```python
from build123d import *

# Parameters (mm, degrees)
SKETCH1_W           = 77.47
SKETCH1_H           = 52.07
SKETCH1_R           = 1.5875
SKETCH1_H_2         = 52.34
BOSS_EXTRUDE3_DEPTH = 6.35
SKETCH2_W           = 19.05
SKETCH2_H           = 1
CUT_EXTRUDE1_DEPTH  = 193.995155978
SKETCH4_W           = 19.05
SKETCH4_H           = 1
CUT_EXTRUDE2_DEPTH  = 193.995155978
SKETCH5_W           = 257.81
SKETCH5_H           = 1
BOSS_EXTRUDE4_DEPTH = 215.9
SKETCH6_W           = 57.15
SKETCH6_H           = 31.75
CUT_EXTRUDE3_DEPTH  = 193.964841955
CUT_EXTRUDE5_DEPTH  = 193.995155978


with BuildPart() as part:
    # Sketch1 → Boss-Extrude3 (new body)
    with BuildSketch(Plane(origin=(0, 0, 0), x_dir=(1, 0, 0), z_dir=(0, 1, 0))):
        Polygon((148.59, 94.11025641), (129.54, 94.11025641), (129.54, 113.16025641), (-137.02974359, 113.16025641), (-137.02974359, 93.98), (-156.21, 93.98), (-156.21, -88.9), (-137.16, -88.9), (-137.16, -106.95), (-156.21, -106.95), (-156.21, -107.95), (148.59, -107.95), (148.59, -106.95), (129.54, -106.95), (129.54, -88.9), (148.59, -88.9), align=None)
        with Locations((-95.885, -80.915)):
            Rectangle(SKETCH1_W, SKETCH1_H, mode=Mode.SUBTRACT)
        with Locations((-5.715, -80.915)):
            Rectangle(SKETCH1_W, SKETCH1_H, mode=Mode.SUBTRACT)
        with Locations((84.455, -80.915)):
            Rectangle(SKETCH1_W, SKETCH1_H, mode=Mode.SUBTRACT)
        with Locations((84.455, 82.915)):
            Rectangle(SKETCH1_W, SKETCH1_H, mode=Mode.SUBTRACT)
        with Locations((84.455, 28.305)):
            Rectangle(SKETCH1_W, SKETCH1_H, mode=Mode.SUBTRACT)
        with Locations((84.455, -26.305)):
            Rectangle(SKETCH1_W, SKETCH1_H, mode=Mode.SUBTRACT)
        with Locations(Location((139.065, 75.334869264, 0), (0, 0, 270))):
            Circle(SKETCH1_R, mode=Mode.SUBTRACT)
        with Locations(Location((139.065, 80.910552749, 0), (0, 0, 270))):
            Circle(SKETCH1_R, mode=Mode.SUBTRACT)
        with Locations(Location((139.065, 86.618990604, 0), (0, 0, 270))):
            Circle(SKETCH1_R, mode=Mode.SUBTRACT)
        with Locations((-5.715, 82.915)):
            Rectangle(SKETCH1_W, SKETCH1_H, mode=Mode.SUBTRACT)
        with Locations((-95.885, -26.305)):
            Rectangle(SKETCH1_W, SKETCH1_H, mode=Mode.SUBTRACT)
        with Locations((-5.715, -26.17)):
            Rectangle(SKETCH1_W, SKETCH1_H_2, mode=Mode.SUBTRACT)
        with Locations((-95.885, 28.305)):
            Rectangle(SKETCH1_W, SKETCH1_H, mode=Mode.SUBTRACT)
        with Locations((-5.715, 28.305)):
            Rectangle(SKETCH1_W, SKETCH1_H, mode=Mode.SUBTRACT)
        with Locations((-95.885, 82.915)):
            Rectangle(SKETCH1_W, SKETCH1_H, mode=Mode.SUBTRACT)
    extrude(amount=BOSS_EXTRUDE3_DEPTH)

    # Sketch2 → Cut-Extrude1 (cut, through all)
    with BuildSketch(Plane(origin=(0, 6.35, 0), x_dir=(1, 0, 0), z_dir=(0, 1, 0))):
        with Locations((139.065, -107.45)):
            Rectangle(SKETCH2_W, SKETCH2_H)
    extrude(amount=-CUT_EXTRUDE1_DEPTH, mode=Mode.SUBTRACT)

    # Sketch4 → Cut-Extrude2 (cut, through all)
    with BuildSketch(Plane(origin=(0, 6.35, 0), x_dir=(1, 0, 0), z_dir=(0, 1, 0))):
        with Locations((-146.685, -107.45)):
            Rectangle(SKETCH4_W, SKETCH4_H)
    extrude(amount=-CUT_EXTRUDE2_DEPTH, mode=Mode.SUBTRACT)

    # Sketch5 → Boss-Extrude4 (add)
    with BuildSketch(Plane.XY.offset(-108.95)):
        with Locations((-5.715, 0.5)):
            Rectangle(SKETCH5_W, SKETCH5_H)
    extrude(amount=BOSS_EXTRUDE4_DEPTH)

    # Sketch6 → Cut-Extrude3 (cut, through all)
    with BuildSketch(Plane(origin=(0, 1, 0), x_dir=(1, 0, 0), z_dir=(0, 1, 0))):
        with Locations((-95.885, 82.915)):
            Rectangle(SKETCH6_W, SKETCH6_H)
        with Locations((-95.885, 28.305)):
            Rectangle(SKETCH6_W, SKETCH6_H)
        with Locations((-95.885, -26.305)):
            Rectangle(SKETCH6_W, SKETCH6_H)
        with Locations((-95.885, -80.915)):
            Rectangle(SKETCH6_W, SKETCH6_H)
        with Locations((-5.715, 82.915)):
            Rectangle(SKETCH6_W, SKETCH6_H)
        with Locations((84.455, 82.915)):
            Rectangle(SKETCH6_W, SKETCH6_H)
        with Locations((-5.715, 28.305)):
            Rectangle(SKETCH6_W, SKETCH6_H)
        with Locations((-5.715, -26.305)):
            Rectangle(SKETCH6_W, SKETCH6_H)
        with Locations((-5.715, -80.915)):
            Rectangle(SKETCH6_W, SKETCH6_H)
        with Locations((84.455, -80.915)):
            Rectangle(SKETCH6_W, SKETCH6_H)
        with Locations((84.455, -26.305)):
            Rectangle(SKETCH6_W, SKETCH6_H)
        with Locations((84.455, 28.305)):
            Rectangle(SKETCH6_W, SKETCH6_H)
    extrude(amount=-CUT_EXTRUDE3_DEPTH, mode=Mode.SUBTRACT)

    # Sketch7 → Cut-Extrude5 (cut, through all)
    with BuildSketch(Plane(origin=(0, 6.35, 0), x_dir=(1, 0, 0), z_dir=(0, 1, 0))):
        Polygon((39.37, 43.846772262), (35.788770068, 40.26554233), (42.679389728, 33.37492267), (35.788770068, 26.48430301), (42.679389728, 19.593683351), (39.37, 16.284293623), (35.788770068, 12.703063691), (42.679389728, 5.812444031), (35.788770068, -1.078175628), (42.679389728, -7.968795288), (35.788770068, -14.859414948), (39.37, -18.44064488), (42.679389728, -21.750034608), (35.788770068, -28.640654267), (42.679389728, -35.531273927), (39.37, -38.840663655), (39.37, -107.95), (-160.951266418, -107.95), (-160.951266418, 113.16025641), (39.37, 113.16025641), align=None)
    extrude(amount=-CUT_EXTRUDE5_DEPTH, mode=Mode.SUBTRACT)


solid = part.part
```
Can you work these out from the model? Positions are in its coordinate system, mm. A direction names the side the tool comes from. Give positions to 0.01 mm unless a question says otherwise; leave off trailing zeros. Loops run counter-clockwise (first coordinate to the right, second up) from the corner with the lowest first, then second, coordinate; pieces in that order, holes last. Notation, with made-up numbers: M 34,32.25 L 54,32.25 A27 ccw 54,69.25 Z; hole C -19,71.25 d5. An arc over 180 degrees is marked long. Use CSV: the item, a comma, the result in double quotes. Start each with the question number.
1. On a 3-axis mill with a long thin cutter (end or side, diameter ignored), from which of +Z, -Z, +X, -X, +Y, -Y can I reach the whole of each face in a straight line? I mean faces 4 (the face through (84, 4, 0.27)), 5 (the face through (39.186, 3.219, -36.868)). Say none if no direction works.
2. If I drill on L1, parallel to Z at x = 106.5, y = 4.25; L2, parallel to X at y = 2.75, z = 83; L3, parallel to X at y = 3.75, z = 25.5, over which ranges is the centre line in solid material (lowest first)?
3. Imagine slicing it at D-D, the plane x = 68. Count the separate pieces of the cut face and the enclosed holes in it, plus the area to 3 significant figures.
4. Imagine slicing it at A-A, the plane z = 67.5. Write out the boundary of the cut face in (x, y).
5. Imagine slicing it at C-C, the plane z = -52. Write out the boundary of the cut face in (x, y).
6. Imagine slicing it at B-B, the plane x = 51. Write out the boundary of the cut face in (y, z).
7. For P1, Ø3, axis at x = 139.5, y = 2.5, coming from the -Z side; P2, Ø0.8, axis at y = 0.5, z = -27, coming from the -X side; P3, Ø10, axis at x = 107, z = -60.5, coming from the -Y side; P4, Ø1.9, axis at x = 141.5, y = 2.5, coming from the +Z side, each with a flat end and sliding along its axis, tell me the tip position at first contact or that it passes through.
8. If we mould it in two halves opening along Z, with no side actions, what happens to faces 1 (the face through (84, 1, -46)), 2 (the face through (139, 3, 88.9)), 3 (the face through (129.54, 3, -104))? For each: released by +Z, released by -Z, zero draft, split by the parting line, or undercut.
Response values:
1,face 4,"+Y"
1,face 5,"-X, +Y, -Y"
2,L1,"-113.16 to -108.95, -56.88 to -54.34, -2.27 to 0.27, 52.34 to 54.88, 106.95 to 107.95"
2,L2,"39.37 to 45.72, 123.19 to 148.59"
2,L3,"38.93 to 45.72, 123.19 to 148.59"
3,separate pieces,"5"
3,enclosed holes,"0"
3,area,"163 mm^2"
4,outline,"M 39.37,0 L 55.88,0 L 55.88,1 L 45.72,1 L 45.72,6.35 L 39.37,6.35 Z; M 113.03,0 L 148.59,0 L 148.59,6.35 L 123.19,6.35 L 123.19,1 L 113.03,1 Z"
5,outline,"M 39.37,0 L 148.59,0 L 148.59,6.35 L 123.19,6.35 L 123.19,1 L 45.72,1 L 45.72,6.35 L 39.37,6.35 Z"
6,outline,"M 0,-113.16 L 6.35,-113.16 L 6.35,-108.95 L 1,-108.95 L 1,-56.88 L 6.35,-56.88 L 6.35,-54.34 L 1,-54.34 L 1,-2.27 L 6.35,-2.27 L 6.35,0.27 L 1,0.27 L 1,52.34 L 6.35,52.34 L 6.35,54.88 L 1,54.88 L 1,106.95 L 6.35,106.95 L 6.35,107.95 L 0,107.95 Z"
7,P1,"z = -94.11"
7,P2,"x = 35.9"
7,P3,"y = 0"
7,P4,"z = 88.9"
8,face 1,"undercut"
8,face 2,"released by +Z"
8,face 3,"zero draft"
